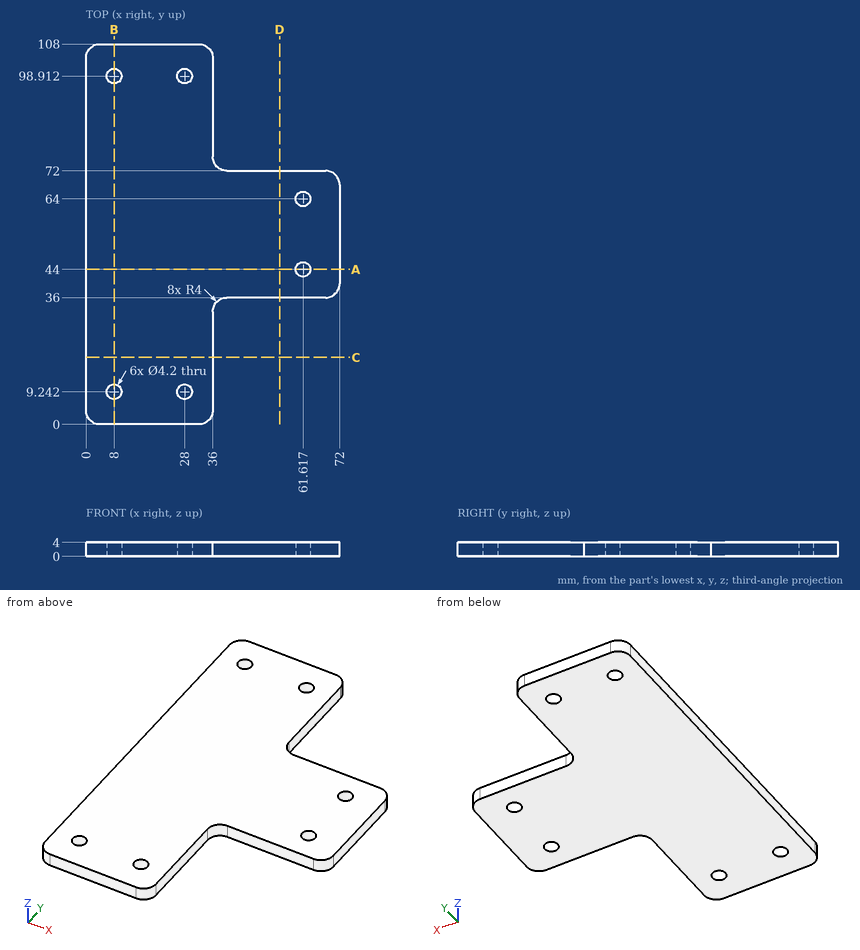
Input: dimensioned drawing with shaded views. Units: mm. Origin: part minimum x, y, z. Coordinates: 2 decimals unless noted, no trailing zeros. Loops run counter-clockwise (first coordinate to the right, second up) from the corner with the lowest first, then second, coordinate; pieces in that order, holes last.
Q1. Section D-D, the plane x = 55. Return the cut outline in (y, z).
Results are:
outline: (36, 0) - (72, 0) - (72, 4) - (36, 4) - close
Q2. Contact query for flat-ended pins moving along their axis: pin 1 (1.5 mm diameter, centred on x = 46.5, z = 3.5, fed in from +Y); pin 2 (5.5 mm diameter, centred on x = 8, y = 98.91, fed in from +Z). Output: stop coordinate, or through.
Results are:
pin 1: stops at y = 72
pin 2: stops at z = 4
Q3. Section C-C, the plane y = 19. Return the cut outline in (x, z), and give its area (3 significant figures).
Results are:
outline: (0, 0) - (36, 0) - (36, 4) - (0, 4) - close
area: 144 mm2
Q4. Line query: line 1 along Y through (x, z) = (8, 2.5); line 2 along Y through (x, z) = (9.5, 1.25) (1 decimal); line 3 along X through (y, z) = (11, 2.75). Output: solid intervals per line, ascending.
Results are:
line 1: y = 0 to 7.14, 11.34 to 96.81, 101.01 to 108
line 2: y = 0 to 7.8, 10.7 to 97.4, 100.4 to 108
line 3: x = 0 to 6.85, 9.15 to 26.85, 29.15 to 36
Q5. Section A-A, the plane y = 44. Return the cut outline in (x, z).
Results are:
outline: (0, 0) - (59.52, 0) - (59.52, 4) - (0, 4) - close; (63.72, 0) - (72, 0) - (72, 4) - (63.72, 4) - close
Q6. Section B-B, the plane x = 8. Return the cut outline in (y, z).
Results are:
outline: (0, 0) - (7.14, 0) - (7.14, 4) - (0, 4) - close; (11.34, 0) - (96.81, 0) - (96.81, 4) - (11.34, 4) - close; (101.01, 0) - (108, 0) - (108, 4) - (101.01, 4) - close
